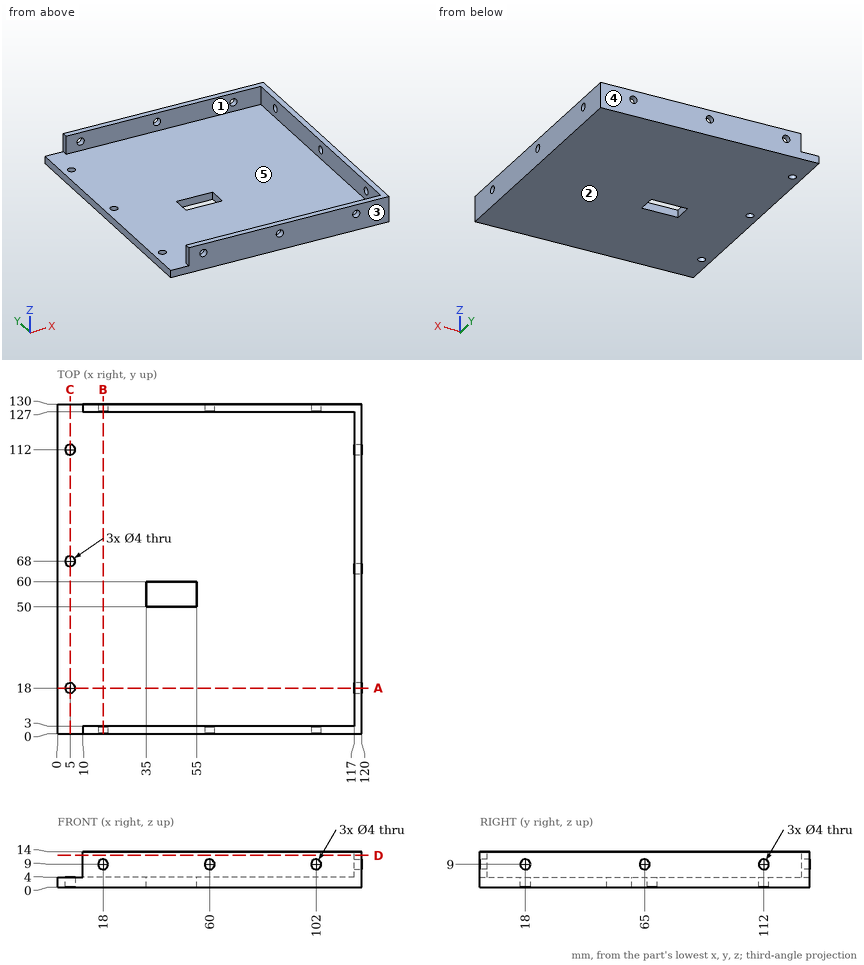
Input: dimensioned drawing with shaded views. Units: mm. Origin: part minimum x, y, z. A direction names the side the tool comes from. Give positions to 0.01 mm unless a question says otherwise; leave off trailing zeros. Order: outer loops, then holes, each group sorted by start corner. A loop starts at its lowest first (then second) coordinate and runs counter-clockwise, first axis right, second up.
(1) Section query B-B (x = 18). Return the cut outline in (y, z).
(2) Material intervals for line 1 along Y through (x, z) = (26.5, 7); line 2 along Z through (x, y) = (18, 1.2); line 3 along Z through (x, y) = (68.5, 40), sorted ascending.
(3) Section query C-C (x = 5). Return the cut outline in (y, z).
(4) Contact query for flat-ended pins moving along their axis: P1, Ø5, axis at y = 68.5, z = 12, coming from the -X side; P2, Ø6.5, axis at x = 5, y = 68, coming from the +Z side; P3, Ø2.5, axis at y = 1.5, z = 8, coming from the -X side; P4, Ø6, axis at x = 17, z = 10, coming from the -Y side. Output: stop coordinate, or through.
(5) Section query A-A (y = 18). Return the cut outline in (x, z).
(6) Section query D-D (z = 12.5). Return the cut outline in (x, y).
(7) Access query for the marked faces 1 and 2. Directions: +Z, -Z, +X, -X, +Y, -Y. A direction counts if a zero-diameter tool reaches every point of the face in a straight line with its end or side. Return the directions, or none.
(8) Pull-direction query (Y, two-part tool) for the marked faces 3, 4 and 5; classes: +Y half, -Y half, draft (parallel to the pull), parting line (faces both ways), or undercut.
Outcome:
1. outline: (0, 0) - (130, 0) - (130, 7) - (127, 7) - (127, 4) - (3, 4) - (3, 7) - (0, 7) - close; (0, 11) - (3, 11) - (3, 14) - (0, 14) - close; (127, 11) - (130, 11) - (130, 14) - (127, 14) - close
2. line 1: y = 0 to 3, 127 to 130
2. line 2: z = 0 to 7, 11 to 14
2. line 3: z = 0 to 4
3. outline: (0, 0) - (16, 0) - (16, 4) - (0, 4) - close; (20, 0) - (66, 0) - (66, 4) - (20, 4) - close; (70, 0) - (110, 0) - (110, 4) - (70, 4) - close; (114, 0) - (130, 0) - (130, 4) - (114, 4) - close
4. P1: stops at x = 117
4. P2: stops at z = 4
4. P3: stops at x = 10
4. P4: stops at y = 0
5. outline: (0, 0) - (3, 0) - (3, 4) - (0, 4) - close; (7, 0) - (120, 0) - (120, 7) - (117, 7) - (117, 4) - (7, 4) - close; (117, 11) - (120, 11) - (120, 14) - (117, 14) - close
6. outline: (10, 0) - (120, 0) - (120, 130) - (10, 130) - (10, 127) - (117, 127) - (117, 3) - (10, 3) - close
7. face 1: +Z, -X
7. face 2: -Z, +X, -X, +Y, -Y
8. face 3: -Y half
8. face 4: +Y half
8. face 5: undercut
